Model file for the job. Use its own axes, mm. Round coordinates to 2 decimals unless told otherwise and drop trailing zeros. Order: outer loops, then holes, each group sorted by start corner. A loop starts at its lowest first (then second) coordinate and runs counter-clockwise, first axis right, second up. Notation, with made-up numbers: (-34.75, 33) - (-1.75, 33) arc R23 cw to (-1.75, 72) - close; hole circle Ø6 at (24, 80). An arc over 180 degrees is marked (long way). Write item = value, one per line. Start each with the question number.
Autodesk Inventor part; units mm, degrees
ref_plane "YZ Plane" through (0, 0, 0) normal (1, 0, 0) x (0, 1, 0)
ref_plane "XZ Plane" through (0, 0, 0) normal (0, 1, 0) x (-1, 0, 0)
ref_plane "XY Plane" through (0, 0, 0) normal (0, 0, 1) x (1, 0, 0)
sketch "Sketch1" plane through (0, 0, 0) normal (0, 0, 1) x (1, 0, 0)
  circle A0 centre (-7.9941, -76.1042) radius 50.9
  line L0 (42.9059, -433.1479) -> (-58.8941, -433.1479)
  arc A1 (-58.8941, -127.0042) -> (42.9059, -127.0042) centre (-7.9941, -76.1042) ccw
  line L1 (147.9059, -76.1042) -> (147.9059, -176.1042)
  line L2 (147.9059, -176.1042) -> (42.9059, -176.1042)
  line L3 (42.9059, -176.1042) -> (42.9059, -127.0042)
  line L4 (-58.8941, -176.1042) -> (-163.8941, -176.1042)
  line L5 (-163.8941, -176.1042) -> (-163.8941, -76.1042)
  line L6 (-163.8941, -76.1042) -> (-58.8941, -76.1042)
  line L7 (-58.8941, -76.1042) -> (-58.8941, -176.1042)
  line L8 (-58.8941, -176.1042) -> (42.9059, -176.1042)
  line L9 (-33.8941, -143.2668) -> (-33.8941, -176.1042)
  arc A2 (147.9059, -76.1042) -> (-163.8941, -76.1042) centre (-7.9941, -76.1042) ccw
  line L10 (-58.8941, -180.1042) -> (-167.8941, -180.1042)
  line L11 (-167.8941, -180.1042) -> (-167.8941, -76.1042)
  line L12 (-58.8941, -180.1042) -> (42.9059, -180.1042)
  line L13 (42.9059, -180.1042) -> (151.9059, -180.1042)
  line L14 (151.9059, -180.1042) -> (151.9059, -76.1042)
  arc A3 (151.9059, -76.1042) -> (-167.8941, -76.1042) centre (-7.9941, -76.1042) ccw
  line L15 (-58.8941, 79.7958) -> (-188.8941, 79.7958)
  line L16 (-188.8941, 79.7958) -> (-188.8941, -50.2042)
  line L17 (-188.8941, -50.2042) -> (-58.8941, -50.2042)
  line L18 (-58.8941, -50.2042) -> (-58.8941, 79.7958)
  line L19 (-58.8941, -76.1042) -> (-58.8941, -50.2042)
  line L20 (-58.8941, -176.1042) -> (-58.8941, -180.6362)
  line L21 (-58.8941, 79.7958) -> (-7.9941, 79.7958)
  line L22 (-188.8941, 79.7958) -> (-7.9941, 79.7958)
  line L23 (-7.9941, 79.7958) -> (-7.9941, 83.7958)
  line L24 (-7.9941, 83.7958) -> (-188.8941, 83.7958)
  line L25 (-188.8941, 83.7958) -> (-188.8941, 79.7958)
  point P0 (0, 0)
  dimension "d0" = 101.8
  dimension "d2" = 100
  dimension "d3" = 130
  dimension "d4" = 4
  dimension "d5" = 4
  dimension "d6" = 4
  dimension "d18" = 130
  dimension "d19" = 130
extrude "Extrusion4" add sketch "Sketch1" along normal blind 4 contours A0 | L19 L18 A2 L1 L2 L3 A1 L7 | A1 L9 L8 L7 | L17 A2 L18 | L17 A3 L18 A2 | A1 L3 L8 L9 | L8 L2 L1 A2 L23 A3 L14 L13 L12 L20 | L18 A3 L21 A2 | L17 L16 L15 L18 A3 | L21 A3 L23 | L18 L21 A3 | L21 L15 L25 L24 A3
equation "\"d20\" = d5"
properties part number "Shooter"
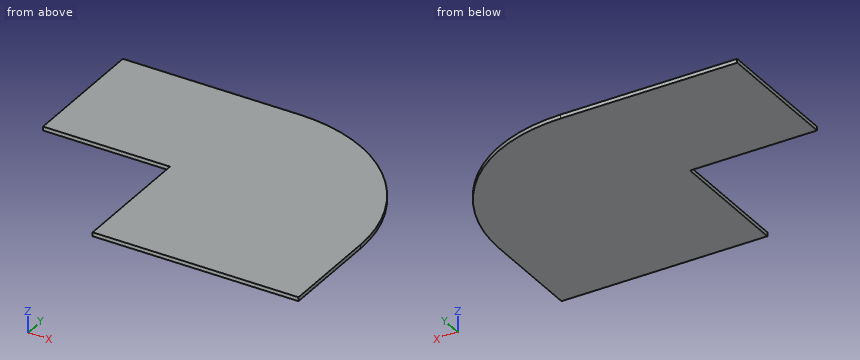
Item 1: Saw through at C-C, the plane y = -117.5. Give the cut face in (x, z), then the cut area to 3 significant figures.
Item 2: Saw through at A-A, the plane z = 2.2. Give the cut face in (x, y).
Item 3: Probe L1, parallel to X at y = -166, z = 0.45; L2, parallel to Y at x = -65, z = 1.35; L3, parallel to Y at x = 69, z = 3.5. List the from-to ranges inside material, lowest first.
Item 4: Saw through at B-B, the plane x = -150. Give the cut face in (y, z), then the cut area to 3 significant figures.
Check sheet entries:
q1.outline = (-58.89, 0) - (151.91, 0) - (151.91, 4) - (-58.89, 4) - close
q1.area = 843 mm2
q2.outline = (-188.89, -50.2) - (-58.89, -50.2) - (-58.89, -180.1) - (151.91, -180.1) - (151.91, -76.1) arc R159.9 ccw to (-7.99, 83.8) - (-188.89, 83.8) - close
q3.L1 = -58.89 to 151.91
q3.L2 = -50.2 to 83.8
q3.L3 = -180.1 to 64.04
q4.outline = (-50.2, 0) - (83.8, 0) - (83.8, 4) - (-50.2, 4) - close
q4.area = 536 mm2
